Verification items for the finished model (mm, model axes). A direction names the side the tool comes from. Give positions to 0.01 mm unless a question says otherwise; leave off trailing zeros. Write each loop counter-clockwise with the first axis right and the second up, starting at its lowest first coordinate (ties: lowest second). Pieces come first, ordered by that corner, then holes. Notation, with made-up numbers: (48, 65.5) -> (53, 65.5) arc R11 ccw to (53, 69.5) -> close; hole circle Ø8 at (62.5, 10). An arc over 180 degrees is marked (long way). Use one line per item in the form item = value. Start each with the question number.
(1) Section check D-D, the plane y = -1.5. Record the cut outline in (x, z).
(2) Section check B-B, the plane z = -14. Record the cut outline in (x, y) (3 decimals), plus the area to 3 significant figures.
(3) Depth check by flat-ended pin: pin 1 Ø10 at (x, z) = (-7.5, 4) entering from +Y; pin 2 Ø1.9 at (x, y) = (-14.5, -3) entering from +Z; pin 3 Ø2 at (y, z) = (-3, 5) entering from -X; pin 4 Ø1 at (x, y) = (4, -4.5) entering from -Z. Enter the tip coordinate at first touch or a pass-through.
(4) Release check for a two-part mould opening along Z. For faces 1 (the face through (-14.29, -3.13, 2.13)), 2 (the face through (-0.413, -6.323, -15.997)), 3 (the face through (2.46, -3.13, 14.04)), 4 (the face through (-9.569, -3.131, -15.206)) record: pulls with the +Z half, pulls with the -Z half, needs draft (parallel to the pull), parting line crosses it, or undercut.
(5) Section check A-A, the plane y = -5.5. Record the cut outline in (x, z), plus the area to 3 significant figures.
(6) Set-up check for faces 5 (the face through (-13, -3, 6.677)), 6 (the face through (5, -3, -12.867)), 7 (the face through (9.48, -3.13, -15.14)): record each of +Z, -Z, +X, -X, +Y, -Y from which the full face is reachable in a straight line by a thin tool's end or side.
(7) Scan lines: L1, parallel to X at y = -2.75, z = -14.5; L2, parallel to Z at x = -6, y = -4.25; L3, parallel to X at y = -2.25, z = 0.5. Record each from-to range of solid material in increasing order.
(8) Section check C-C, the plane x = 2. Record the cut outline in (y, z), plus the area to 3 significant figures.
from build123d import *

# Parameters (mm, degrees)
F1_DEPTH = 6.35
F2_R     = 3.175
F3_DEPTH = 6.35


with BuildPart() as f1:
    # F0 (on Front) → F1 (new body)
    with BuildSketch(Plane.XZ):
        Polygon((4.850968, 6.676785), (0, 21.606531), (-4.850968, 6.676785), (-20.549032, 6.676785), (-7.849032, -2.550305), (-12.7, -17.48005), (-6.35, -12.866505), (6.35, -12.866505), (12.7, -17.48005), (7.849032, -2.550305), (20.549032, 6.676785), align=None)
    extrude(amount=F1_DEPTH)

    # F2 (on face) → F3 (join)
    with BuildSketch(Plane(origin=(0, 0, -12.866505), x_dir=(1, 0, 0), z_dir=(0, 0, -1))):
        with Locations((0, 3.175)):
            Circle(F2_R)
    extrude(amount=F3_DEPTH)


solid = f1.part
Completed:
q1.outline = (-20.55, 6.68) -> (-7.85, -2.55) -> (-12.7, -17.48) -> (-6.35, -12.87) -> (-2.7, -12.87) -> (-2.7, -19.22) -> (2.7, -19.22) -> (2.7, -12.87) -> (6.35, -12.87) -> (12.7, -17.48) -> (7.85, -2.55) -> (20.55, 6.68) -> (4.85, 6.68) -> (0, 21.61) -> (-4.85, 6.68) -> close
q2.outline = (-11.569, -6.35) -> (-7.91, -6.35) -> (-7.91, 0) -> (-11.569, 0) -> close; circle Ø6.35 at (0, -3.175); (7.91, -6.35) -> (11.569, -6.35) -> (11.569, 0) -> (7.91, 0) -> close
q2.area = 78.1 mm²
q3.pin_1 = 0
q3.pin_2 = 6.68
q3.pin_3 = -19.62
q3.pin_4 = -12.87
q4.face_1 = undercut
q4.face_2 = needs draft
q4.face_3 = pulls with the +Z half
q4.face_4 = pulls with the -Z half
q5.outline = (-20.55, 6.68) -> (-7.85, -2.55) -> (-12.7, -17.48) -> (-6.35, -12.87) -> (-2.16, -12.87) -> (-2.16, -19.22) -> (2.16, -19.22) -> (2.16, -12.87) -> (6.35, -12.87) -> (12.7, -17.48) -> (7.85, -2.55) -> (20.55, 6.68) -> (4.85, 6.68) -> (0, 21.61) -> (-4.85, 6.68) -> close
q5.area = 581 mm²
q6.face_5 = +Z, -X, +Y, -Y
q6.face_6 = -Z
q6.face_7 = -Z, +Y, -Y
q7.L1 = -11.73 to -8.6, -3.15 to 3.15, 8.6 to 11.73
q7.L2 = -12.87 to 6.68
q7.L3 = -12.05 to 12.05
q8.outline = (-6.35, -12.87) -> (-5.64, -12.87) -> (-5.64, -19.22) -> (-0.71, -19.22) -> (-0.71, -12.87) -> (0, -12.87) -> (0, 15.45) -> (-6.35, 15.45) -> close
q8.area = 211 mm²
